CAD build for the part. Positions are in the model's coordinates, mm. Round coordinates to 2 decimals unless told otherwise and drop trailing zeros. Order: outer loops, then holes, each group sorted by start corner. A loop starts at its lowest first (then second) coordinate and runs counter-clockwise, first axis right, second up. Notation, with made-up numbers: (77.25, -1.5) -> (111.25, -1.5) arc R24 ccw to (111.25, 13.5) -> close; hole circle Ø3 at (22.25, -21.75). An arc over 180 degrees is marked (long way). Answer as CSV lines item,"result". Start each with the question number.
from build123d import *

# Parameters (mm, degrees)
F0_R     = 57
F2_DEPTH = 50
F4_R     = 10


with BuildPart() as f2:
    # F0 (on Top) → F2 (new body)
    with BuildSketch(Plane.XY):
        Circle(F0_R)
    extrude(amount=F2_DEPTH)

    # F1 (on Front) → F3 (revolve, cut)
    with BuildSketch(Plane.XZ):
        with BuildLine():
            Line((0, 100.7613007724), (0, 20.7613007724))
            ThreePointArc((0, 20.7613007724), (40, 60.7613007724), (0, 100.7613007724))
        make_face()
    revolve(axis=Axis((0, 0, 40.7613007724), (0, 0, -1)), mode=Mode.SUBTRACT)

    # F4
    f4_edges = [f2.edges().sort_by_distance(p)[0] for p in [
        (-57, 0, 50),
        (-38.525244, 0, 50),
    ]]
    fillet(f4_edges, radius=F4_R)


solid = f2.part
Item 1: Probe line 1 (Y direction, x = 22.5, z = 34.5); line 2 (X direction, y = 17.5, z = 37); line 3 (Y direction, x = 18.5, z = 37). List the from-to ranges inside material, lowest first.
Item 2: Band-saw the part on A-A, the plane z = 26. Give the cut face in (x, y), and give its area (3 significant figures).
Item 3: Pin check, flat tips, straight feed: pin 1 (10 mm diameter, centred on x = 24.5, z = 9.5, fed in from +Y); pin 2 (4 mm diameter, centred on x = 42, z = 23.5, fed in from -Y); pin 3 (1.5 mm diameter, centred on x = 9, z = 15, fed in from -Y). Stop position of each tip, or through.
Item 4: Band-saw the part on B-B, the plane z = 5. Give the cut face in (x, y), and give its area (3 significant figures).
Values:
1,line 1,"-52.37 to -20.1, 20.1 to 52.37"
1,line 2,"-54.25 to -27, 27 to 54.25"
1,line 3,"-53.91 to -26.33, 26.33 to 53.91"
2,outline,"circle Ø114 at (0, 0); hole circle Ø39.58 at (0, 0)"
2,area,"8,980 mm²"
3,pin 1,"y = 53.56"
3,pin 2,"y = -40.61"
3,pin 3,"y = -56.4"
4,outline,"circle Ø114 at (0, 0)"
4,area,"10,200 mm²"
